Input: part model. Units: mm. Frame: model coordinates. A direction names the side the tool comes from. Round coordinates to 2 decimals unless told otherwise and drop trailing zeros. Loops run counter-clockwise (first coordinate to the right, second up) from the corner with the lowest first, then second, coordinate; pieces in that order, holes last.
1) Section B-B, the plane z = 3.2. State how many separate pieces and enclosed holes the cut face has, and give its area (3 significant figures).
2) Section D-D, the plane y = 23.5. Return loops of the section in (x, z).
3) Draft query along Y for faces 4 (the face through (-5.55, 26, 3)), 5 (the face through (45, 29.5, 1)), 6 (the face through (-0.409, -11.493, 3.155)). Return one class per face: pulls with the +Y half, pulls with the -Y half, needs draft (parallel to the pull), parting line crosses it, or undercut.
4) Section C-C, the plane y = 41. Return loops of the section in (x, z), and give its area (3 significant figures).
5) Ray query, line 1 along Y through (x, z) = (0, 4.25); line 2 along X through (y, z) = (14.5, 1.5); line 3 along Y through (x, z) = (24, 1.5). Return the intervals inside material, ascending.
6) Section A-A, the plane y = 0. Return loops of the section in (x, z), and give its area (3 significant figures).
7) Access query for faces 1 (the face through (6.19, 33.27, 3.24)), 2 (the face through (45, 27, 1.55)), 3 (the face through (-5.8, 10.29, 3.24)). Directions: +Z, -Z, +X, -X, +Y, -Y. A direction counts if a zero-diameter tool reaches every point of the face in a straight line with its end or side. Return the directions, or none.
8) First-contact query: pin 1 (3 mm diameter, centred on x = 44.5, z = 3.5, fed in from +Y); pin 2 (1.5 mm diameter, centred on y = 16.5, z = 5.5, fed in from +X); pin 3 (8 mm diameter, centred on x = 0, y = 0, fed in from +Z); pin 4 (3 mm diameter, centred on x = 42.5, z = 2.5, fed in from -Y). Flat tips, straight axial feed; report the tip coordinate or a pass-through.
from build123d import *

# Parameters (mm, degrees)
SKETCH1_R           = 2.55
SKETCH1_R_2         = 8.07
BOSS_EXTRUDE3_DEPTH = 6.4
CUT_EXTRUDE1_DEPTH  = 16
FILLET1_R           = 2.5
FILLET2_R           = 2.25


with BuildPart() as part:
    # Sketch1 → Boss-Extrude3 (new body)
    with BuildSketch(Plane.XY):
        with BuildLine():
            ThreePointArc((-5.55, 10.072114972), (0, -11.5), (5.55, 10.072114972))
            Line((5.55, 10.072114972), (5.55, 33.95))
            Line((5.55, 33.95), (10.604198419, 33.95))
            ThreePointArc((10.604198419, 33.95), (15.944722227, 27.443362824), (24, 25))
            Line((24, 25), (52.5, 25))
            Line((52.5, 25), (52.5, 29.5))
            Line((52.5, 29.5), (34.5, 29.5))
            ThreePointArc((34.5, 29.5), (31.908668769, 51.65331059), (10.604198419, 45.05))
            Line((10.604198419, 45.05), (0, 45.05))
            ThreePointArc((0, 45.05), (-3.924442636, 43.424442636), (-5.55, 39.5))
            Line((-5.55, 39.5), (-5.55, 10.072114972))
        make_face()
        Circle(SKETCH1_R, mode=Mode.SUBTRACT)
        with Locations((24, 39.5)):
            Circle(SKETCH1_R_2, mode=Mode.SUBTRACT)
    extrude(amount=BOSS_EXTRUDE3_DEPTH)

    # Sketch2 → Cut-Extrude1 (cut)
    with BuildSketch(Plane(origin=(0, 29.5, 0), x_dir=(1, 0, 0), z_dir=(0, 1, 0))):
        with BuildLine():
            Line((42.8, -1.55), (47.8, -1.55))
            ThreePointArc((47.8, -1.55), (49.45, -3.2), (47.8, -4.85))
            Line((47.8, -4.85), (42.8, -4.85))
            ThreePointArc((42.8, -4.85), (41.15, -3.2), (42.8, -1.55))
        make_face()
    extrude(amount=-CUT_EXTRUDE1_DEPTH, mode=Mode.SUBTRACT)

    # Fillet1
    fillet1_edges = [part.edges().sort_by_distance(p)[0] for p in [
        (34.5, 29.5, 3.2),
    ]]
    fillet(fillet1_edges, radius=FILLET1_R)

    # Fillet2
    fillet2_edges = [part.edges().sort_by_distance(p)[0] for p in [
        (10.604198419, 33.95, 3.2),
        (-5.55, 10.072114972, 3.2),
        (5.55, 10.072114972, 3.2),
        (5.55, 33.95, 3.2),
        (52.5, 25, 3.2),
        (52.5, 29.5, 3.2),
    ]]
    fillet(fillet2_edges, radius=FILLET2_R - 0.0001)  # a hair under: the kernel refuses the full size


solid = part.part
Final values:
1. separate pieces: 2
1. enclosed holes: 2
1. area: 1,330 mm2
2. outline: (-5.55, 0) - (5.55, 0) - (5.55, 6.4) - (-5.55, 6.4) - close
3. face 4: needs draft
3. face 5: pulls with the +Y half
3. face 6: undercut
4. outline: (-5.34, 0) - (16.07, 0) - (16.07, 6.4) - (-5.34, 6.4) - close; (31.93, 0) - (38.42, 0) - (38.42, 6.4) - (31.93, 6.4) - close
4. area: 179 mm2
5. line 1: y = -11.5 to -2.55, 2.55 to 45.05
5. line 2: x = -5.55 to 5.55
5. line 3: y = 25 to 31.43, 47.57 to 54
6. outline: (-11.5, 0) - (-2.55, 0) - (-2.55, 6.4) - (-11.5, 6.4) - close; (2.55, 0) - (11.5, 0) - (11.5, 6.4) - (2.55, 6.4) - close
6. area: 115 mm2
7. face 1: +Z, -Z
7. face 2: +Y, -Y
7. face 3: +Z, -Z, -X, +Y
8. pin 1: stops at y = 29.5
8. pin 2: stops at x = 5.55
8. pin 3: stops at z = 6.4
8. pin 4: stops at y = 25
